Could you check a few things on this model? Use its own coordinates, in mm. Face numbers are marked on the shaded views. Give positions to 0.01 mm unless a question says otherwise; leave off trailing zeros. Loops run counter-clockwise (first coordinate to the right, second up) from the corner with the lowest first, then second, coordinate; pieces in that order, holes last. Notation, with made-up numbers: (-20.5, 12.25) -> (25.5, 12.25) arc R12 cw to (25.5, 30.25) -> close; hole circle Ø9 at (-23.5, -2.5). An arc over 180 degrees is marked (long way). Put each result on its own line as item: value.
```python
from build123d import *

# Parameters (mm, degrees)
SKETCH1_R           = 12.75
BOSS_EXTRUDE1_DEPTH = 31
SKETCH2_R           = 11.25
CUT_EXTRUDE1_DEPTH  = 31
SKETCH3_W           = 26.062962729
SKETCH3_H           = 13.122907939
CUT_EXTRUDE2_DEPTH  = 31
SKETCH8_W           = 1.5
SKETCH8_H           = 31
BOSS_EXTRUDE3_DEPTH = 4
SKETCH11_R          = 2
CUT_EXTRUDE3_DEPTH  = 2
CUT_EXTRUDE4_START  = -2
SKETCH9_R           = 2
CUT_EXTRUDE4_DEPTH  = 2


with BuildPart() as part:
    # Sketch1 → Boss-Extrude1 (new body)
    with BuildSketch(Plane.XY):
        Circle(SKETCH1_R)
    extrude(amount=-BOSS_EXTRUDE1_DEPTH)

    # Sketch2 → Cut-Extrude1 (cut)
    with BuildSketch(Plane.XY):
        Circle(SKETCH2_R)
    extrude(amount=-CUT_EXTRUDE1_DEPTH, mode=Mode.SUBTRACT)

    # Sketch3 → Cut-Extrude2 (cut)
    with BuildSketch(Plane.XY):
        with Locations((0.281481365, 6.56145397)):
            Rectangle(SKETCH3_W, SKETCH3_H)
    extrude(amount=-CUT_EXTRUDE2_DEPTH, mode=Mode.SUBTRACT)

    # Sketch8 → Boss-Extrude3 (add)
    with BuildSketch(Plane(origin=(0, 0, 0), x_dir=(1, 0, 0), z_dir=(0, 1, 0))):
        with Locations((-12, 15.5)):
            Rectangle(SKETCH8_W, SKETCH8_H)
        with Locations((12, 15.5)):
            Rectangle(SKETCH8_W, SKETCH8_H)
    extrude(amount=BOSS_EXTRUDE3_DEPTH)

    # Sketch11 → Cut-Extrude3 (cut)
    with BuildSketch(Plane.ZY.offset(12.75)):
        with Locations(Location((-15.5, 0.25, 0), (0, 0, 352.819244219))):
            Circle(SKETCH11_R)
    extrude(amount=-CUT_EXTRUDE3_DEPTH, mode=Mode.SUBTRACT)

    # Sketch9 → Cut-Extrude4 (cut)
    with BuildSketch(Plane(origin=(12.75, 0, 0), x_dir=(0, 0, -1), z_dir=(1, 0, 0)).offset(CUT_EXTRUDE4_START)):
        with Locations(Location((15.5, 0.25, 0), (0, 0, 187.180755781))):
            Circle(SKETCH9_R)
    extrude(amount=CUT_EXTRUDE4_DEPTH, mode=Mode.SUBTRACT)


solid = part.part
```
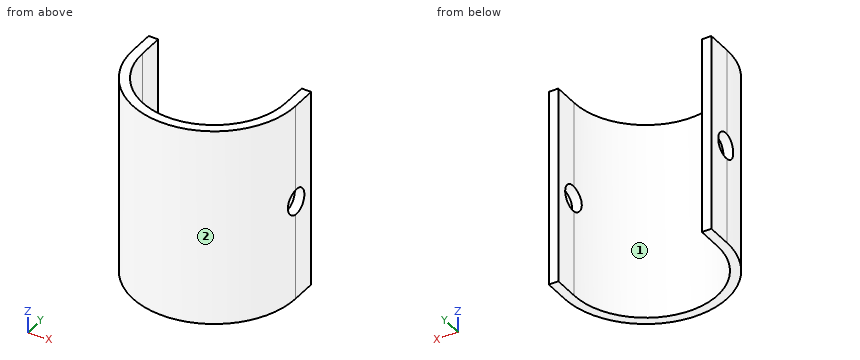
1. If we section it at B-B (y = 0.75): List the corners of the cut face in (x, z) for me.
Recorded:
outline: (-12.75, -31) -> (-11.25, -31) -> (-11.25, -17.44) -> (-12.75, -17.44) -> close; (-12.75, -13.56) -> (-11.25, -13.56) -> (-11.25, 0) -> (-12.75, 0) -> close; (11.25, -31) -> (12.75, -31) -> (12.75, -17.44) -> (11.25, -17.44) -> close; (11.25, -13.56) -> (12.75, -13.56) -> (12.75, 0) -> (11.25, 0) -> close
2. If we section it at D-D (z = -15.5): List the corners of the cut face in (x, y) for me, then the cut area to 3 significant figures.
Recorded:
outline: (-12.75, 2.25) -> (-11.25, 2.25) -> (-11.25, 4) -> (-12.75, 4) -> close; (-12.63, -1.75) arc R12.75 ccw to (12.63, -1.75) -> (11.11, -1.75) arc R11.25 cw to (-11.11, -1.75) -> close; (11.25, 2.25) -> (12.75, 2.25) -> (12.75, 4) -> (11.25, 4) -> close
area: 56.5 mm^2
3. I need wall thicknesses on line 1 (Z direction, x = 12.25, y = 0.25); line 2 (X direction, y = -10.25, z = -3.5); line 3 (X direction, y = 2.5, z = -24). Which ranges of each line are inside material? Lowest first, please.
Recorded:
line 1: z = -31 to -17.5, -13.5 to 0
line 2: x = -7.58 to -4.64, 4.64 to 7.58
line 3: x = -12.75 to -11.25, 11.25 to 12.75
4. I'm going to push flat-ended pins straight in: pin 1 (12 mm diameter, centred on x = -2, z = -14.5, fed in from +Y); pin 2 (1.5 mm diameter, centred on y = -10, z = -18.5, fed in from +X); pin 3 (1.5 mm diameter, centred on x = 5.5, z = -20.5, fed in from +Y). Where does each tip first touch, or does it pass through?
Recorded:
pin 1: stops at y = -7.91
pin 2: stops at x = 8.77
pin 3: stops at y = -9.35
5. If we section it at A-A (y = -8): List the corners of the cut face in (x, z) for me.
Recorded:
outline: (-9.93, -31) -> (-7.91, -31) -> (-7.91, 0) -> (-9.93, 0) -> close; (7.91, -31) -> (9.93, -31) -> (9.93, 0) -> (7.91, 0) -> close
6. Thinking about a two-plate mould opening in X: for the marked faces 1 and 2, which applies, pulls with the +X half, pulls with the -X half, needs draft (parallel to the pull), parting line crosses it, or undercut?
Recorded:
face 1: undercut
face 2: parting line crosses it
7. If we section it at C-C (z = -3): List the corners of the cut face in (x, y) for me.
Recorded:
outline: (-12.75, 0) arc R12.75 ccw to (12.75, 0) -> (12.75, 4) -> (11.25, 4) -> (11.25, 0) arc R11.25 cw to (-11.25, 0) -> (-11.25, 4) -> (-12.75, 4) -> close
